The listing builds one solid part. Answer for the finished solid, in the listing's coordinates (mm). A direction names the side the tool comes from. Coordinates: 2 decimals unless noted, no trailing zeros. Loops run counter-clockwise (first coordinate to the right, second up) from the corner with the lowest first, then second, coordinate; pieces in that order, holes last. Notation, with made-up numbers: (85, 65) - (131, 65) arc R22 ccw to (131, 91) - close; hole circle Ø6 at (23.25, 50.25). An arc over 180 degrees is marked (long way). Write each question's results on one line, items separated by ' | '. Start each with the question number.
(1) For faces 5 (the cylindrical face through (18.696, -15.286, 0.462)), 6 (the flat face through (10, -15, 0)), determine the directions among +Z, -Z, +X, -X, +Y, -Y from which every point of the face is accessible in a straight line to the end or side of a thin tool.
(2) Find section C-C on y = -4.25. Determine the outline of the cut face in (x, z).
(3) Given pin 1 Ø2 at (y, z) = (-4.5, -12) entering from -X; pin 2 Ø2 at (y, z) = (-26, 9.5) entering from +X; pin 3 Ø5 at (x, y) = (7.5, -4) entering from +Z, each flat-ended and moving along its own axis, determine where each tip first touches the part or whether it passes through.
(4) Determine the mould class of faces 1 (the flat face through (36, 0, 0)), 2 (the flat face through (47.69, -14.79, -22.28)), 3 (the cylindrical face through (65.176, -21.051, 0.862)), 4 (the flat face through (0, -15, 5)) for opening direction X: released by +X, released by -X, zero draft, split by the parting line, or undercut.
(5) Consider line 1 (Z direction, x = -5, y = -2); line 2 (X direction, y = -21, z = 11); line 3 (X direction, y = -17.75, z = 11). Determine where each line is inside the solid, lowest interval first. Write a range as from..to.
(6) Find section D-D on z = 0. State how many separate pieces and enclosed holes the cut face has, then the cut area to 3 significant figures.
(7) Find section A-A on x = 0. Determine the outline of the cut face in (y, z), then the cut area to 3 significant figures.
(8) Find section B-B on y = -11.25. Determine the outline of the cut face in (x, z), then the cut area to 3 significant figures.
from build123d import *

# Parameters (mm, degrees)
F1_DEPTH = 30
F2_W     = 20
F2_H     = 10
F3_DEPTH = 30
F4_R     = 6.5
F5_DEPTH = 64.6280276847
F7_D     = 7


with BuildPart() as f1:
    # F0 (on Front) → F1 (new body)
    with BuildSketch(Plane.XZ):
        with BuildLine():
            Line((91.5280898876, 14.7854239547), (5.0561797753, 29.5708479094))
            ThreePointArc((5.0561797753, 29.5708479094), (-30, 0), (5.0561797753, -29.5708479094))
            Line((5.0561797753, -29.5708479094), (91.5280898876, -14.7854239547))
            ThreePointArc((91.5280898876, -14.7854239547), (104, 0), (91.5280898876, 14.7854239547))
        make_face()
    extrude(amount=F1_DEPTH)

    # F2 (on face) → F3 (cut)
    with BuildSketch(Plane.XZ.offset(30)):
        Rectangle(F2_W, F2_H)
    extrude(amount=-F3_DEPTH, mode=Mode.SUBTRACT)

    # F4 (on face) → F5 (cut, through all)
    with BuildSketch(Plane(origin=(5.0561797753, 0, -29.5708479094), x_dir=(0.9856949303, 0, 0.1685393258), z_dir=(0.1685393258, 0, -0.9856949303))):
        with Locations((25, 15)):
            Circle(F4_R)
    extrude(amount=-F5_DEPTH, mode=Mode.SUBTRACT)

    # F7 (through all)
    with Locations(Plane(origin=(5.0561797753, 0, -29.5708479094), x_dir=(0.9856949303, 0, 0.1685393258), z_dir=(0.1685393258, 0, -0.9856949303))):
        with Locations((67.7268487978, 20)):
            Hole(F7_D / 2)


solid = f1.part
Values:
1) face 5: none | face 6: +Y, -Y
2) outline: (5.06, -29.57) - (91.53, -14.79) arc R15 ccw to (91.53, 14.79) - (5.06, 29.57) arc R30 ccw (long way) to start; hole (-10, -5) - (10, -5) - (10, 5) - (-10, 5) - close
3) pin 1: stops at x = -27.91 | pin 2: stops at x = 101.36 | pin 3: stops at z = 29.58
4) face 1: zero draft | face 2: released by +X | face 3: undercut | face 4: undercut
5) line 1: z = -29.58..-5, 5..29.58 | line 2: x = -27.91..20.95, 26.02..63.43, 70.23..99.2 | line 3: x = -27.91..17.51, 29.46..64.11, 69.55..99.2
6) separate pieces: 2 | enclosed holes: 2 | area: 3,250 mm²
7) outline: (-30, -30) - (0, -30) - (0, -5) - (-30, -5) - close; (-30, 5) - (0, 5) - (0, 30) - (-30, 30) - close | area: 1,500 mm²
8) outline: (5.06, -29.57) - (24.47, -26.25) - (15.22, 27.83) - (5.06, 29.57) arc R30 ccw (long way) to start; (26.31, 25.94) - (34.93, -24.46) - (91.53, -14.79) arc R15 ccw to (91.53, 14.79) - close; hole (-10, -5) - (10, -5) - (10, 5) - (-10, 5) - close | area: 5,070 mm²
